from build123d import *

# Parameters (mm, degrees)
F0_W     = 101.6
F0_H     = 127
F1_DEPTH = 25.4
F2_W     = 25.4
F2_H     = 38.1
F3_DEPTH = 25.4
F5_DEPTH = 25.4


with BuildPart() as f1:
    # F0 (on Top) → F1 (new body)
    with BuildSketch(Plane.XY):
        with Locations((3.221489, 1.487175)):
            Rectangle(F0_W, F0_H)
    extrude(amount=F1_DEPTH)

    # F2 (on face) → F3 (join)
    with BuildSketch(Plane.XY.offset(25.4)):
        Polygon((54.021489, 64.987175), (-47.578511, 64.987175), (-47.578511, 26.887175), (-22.178511, 26.887175), (28.621489, 26.887175), (54.021489, 26.887175), align=None)
        with Locations((-34.878511, 7.837175)):
            Rectangle(F2_W, F2_H)
        with Locations((41.321489, 7.837175)):
            Rectangle(F2_W, F2_H)
    extrude(amount=F3_DEPTH)

    # F4 (on face) → F5 (join)
    with BuildSketch(Plane.XY.offset(50.8)):
        Polygon((54.021489, 64.987175), (-47.578511, 64.987175), (-47.578511, 26.887175), (-22.178511, 26.887175), (28.621489, 26.887175), (54.021489, 26.887175), align=None)
    extrude(amount=F5_DEPTH)


solid = f1.part
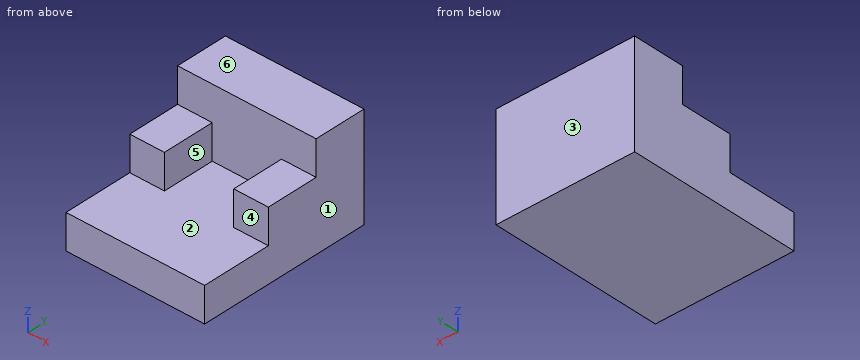
Model file for the job. Use its own axes, mm. Face numbers are marked on the shaded views. A direction names the side the tool comes from. Round coordinates to 2 decimals unless told otherwise and drop trailing zeros. Loops run counter-clockwise (first coordinate to the right, second up) from the corner with the lowest first, then second, coordinate; pieces in that order, holes last. Notation, with made-up numbers: (16, 48) -> (72, 48) arc R19 ccw to (72, 60) -> close; hole circle Ø8 at (32.25, 29.25). An arc over 180 degrees is marked (long way). Answer as CSV lines item,"result". Start each with the question number.
1) Tool access for the marked faces 4, 5 and 6: list every direction of +Z, -Z, +X, -X, +Y, -Y with a clear straight run to the whole face (end or side of a thin tool).
2) Slice it at D-D (x = -13). List the corners of the cut face in (y, z), plus the area to 3 significant figures.
3) Slice it at B-B (z = 46). List the corners of the cut face in (x, y).
4) Slice it at C-C (y = -39). List the corners of the cut face in (x, z).
5) Probe line 1 along X through (y, z) = (18, 36); line 2 along Z through (x, y) = (-40, -33.5); line 3 along Y through (x, z) = (-4.5, 70). List the from-to ranges inside material, lowest first.
6) Slice it at A-A (x = -39). List the corners of the cut face in (y, z).
7) Pin check, flat tips, straight feed: P1, Ø20.5, axis at x = 37, z = 43, coming from the -Y side; P2, Ø7.5, axis at x = -31, y = 1, coming from the +Z side; P3, Ø12, axis at x = -29, z = 64, coming from the -Y side. Stop position of each tip, or through.
8) Mould opens along X. For the marked faces 1, 2 and 3 say: +X half, -X half, draft (parallel to the pull), parting line (faces both ways), or undercut.
Filled in:
1,face 4,"+Z, +X, -X, -Y"
1,face 5,"+Z, -Y"
1,face 6,"+Z, +X, -X, +Y, -Y"
2,outline,"(-62.01, 0) -> (64.99, 0) -> (64.99, 76.2) -> (26.89, 76.2) -> (26.89, 25.4) -> (-62.01, 25.4) -> close"
2,area,"5,160 mm2"
3,outline,"(-47.58, -11.21) -> (-22.18, -11.21) -> (-22.18, 26.89) -> (28.62, 26.89) -> (28.62, -11.21) -> (54.02, -11.21) -> (54.02, 64.99) -> (-47.58, 64.99) -> close"
4,outline,"(-47.58, 0) -> (54.02, 0) -> (54.02, 25.4) -> (-47.58, 25.4) -> close"
5,line 1,"x = -47.58 to -22.18, 28.62 to 54.02"
5,line 2,"z = 0 to 25.4"
5,line 3,"y = 26.89 to 64.99"
6,outline,"(-62.01, 0) -> (64.99, 0) -> (64.99, 76.2) -> (26.89, 76.2) -> (26.89, 50.8) -> (-11.21, 50.8) -> (-11.21, 25.4) -> (-62.01, 25.4) -> close"
7,P1,"stops at y = -11.21"
7,P2,"stops at z = 50.8"
7,P3,"stops at y = 26.89"
8,face 1,"+X half"
8,face 2,"undercut"
8,face 3,"draft"
